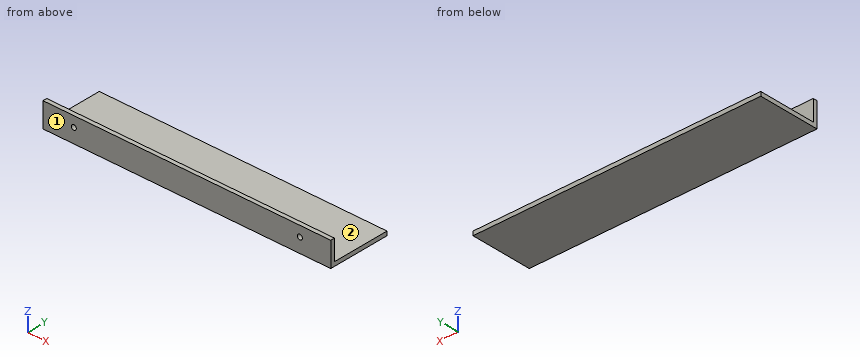
```python
from build123d import *

# Parameters (mm, degrees)
SZKIC1_W                    = 700
SZKIC1_H                    = 150
DODANIE_WYCI_GNI_CIE1_DEPTH = 10
SZKIC2_W                    = 700
SZKIC2_H                    = 10
DODANIE_WYCI_GNI_CIE2_DEPTH = 50
OTW_R_POD_RUB_M101_D        = 12
SZYK_LINIOWY2_COUNT         = 2
SZYK_LINIOWY2_PITCH         = 550


with BuildPart() as part:
    # Szkic1 → Dodanie-wyciągnięcie1 (new body)
    with BuildSketch(Plane.XY):
        Rectangle(SZKIC1_W, SZKIC1_H)
    extrude(amount=DODANIE_WYCI_GNI_CIE1_DEPTH)

    # Szkic2 → Dodanie-wyciągnięcie2 (add)
    with BuildSketch(Plane.XY.offset(10)):
        with Locations((0, -70)):
            Rectangle(SZKIC2_W, SZKIC2_H)
    extrude(amount=DODANIE_WYCI_GNI_CIE2_DEPTH)

    # Otwór pod śrubę M101 (through all)
    with Locations(Plane(origin=(0, -65, 0), x_dir=(1, 0, 0), z_dir=(0, 1, 0))):
        with Locations((-275, -35)):
            otw_r_pod_rub_m101 = Hole(OTW_R_POD_RUB_M101_D / 2)

    # Szyk liniowy2: Otwór pod śrubę M101 ×2
    with Locations(*[(i * SZYK_LINIOWY2_PITCH, 0, 0) for i in range(1, SZYK_LINIOWY2_COUNT)]):
        add(otw_r_pod_rub_m101, mode=Mode.SUBTRACT)


solid = part.part
```
Part model, mm, in its own coordinate system. Face numbers are marked on the shaded views. A direction names the side the tool comes from. Give positions to 0.01 mm unless a question says otherwise; leave off trailing zeros. Write each loop counter-clockwise with the first axis right and the second up, starting at its lowest first coordinate (ties: lowest second). Pieces come first, ordered by that corner, then holes. Notation, with made-up numbers: (-39, 72.25) -> (16, 72.25) arc R9 ccw to (16, 86.25) -> close; hole circle Ø9 at (-33.5, 63). An arc over 180 degrees is marked (long way). Put each result on its own line as item: value. Start each with the question number.
Item 1: Which spindle directions (+Z, -Z, +X, -X, +Y, -Y) get a long thin tool onto all of the face, cutting with end or side? Do the marked faces 1 and 2. Say none if no direction does.
Item 2: Cut at B-B (z = 35). List the corners of the cut face in (x, y), then the cut area to 3 significant figures.
Item 3: Wall check: L1, parallel to Z at x = 275, y = -67.75; L2, parallel to X at y = -69, z = 35; L3, parallel to Y at x = -83, z = 43.5. Give the ranges that are in metal, low to high. Write a range as [from, to].
Item 4: Cut at A-A (x = -275). List the corners of the cut face in (y, z), then the cut area to 3 significant figures.
Item 5: Cut at C-C (y = -7). List the corners of the cut face in (x, z).
Item 6: Cut at D-D (x = 38). List the corners of the cut face in (y, z).
Item 7: Pin check, flat tips, straight feed: pin 1 Ø25 at (x, z) = (-147, 31.5) entering from +Y; pin 2 Ø5 at (y, z) = (15.5, 13.5) entering from -X; pin 3 Ø1.5 at (x, y) = (-227, -13.5) entering from +Z. Stop position of each tip, or through.
Answer list:
1. face 1: +Z, -Z, +X, -X, -Y
1. face 2: +Z, +X, -X, +Y
2. outline: (-350, -75) -> (-281, -75) -> (-281, -65) -> (-350, -65) -> close; (-269, -75) -> (269, -75) -> (269, -65) -> (-269, -65) -> close; (281, -75) -> (350, -75) -> (350, -65) -> (281, -65) -> close
2. area: 6,760 mm2
3. L1: z = [0, 29], [41, 60]
3. L2: x = [-350, -281], [-269, 269], [281, 350]
3. L3: y = [-75, -65]
4. outline: (-75, 0) -> (75, 0) -> (75, 10) -> (-65, 10) -> (-65, 29) -> (-75, 29) -> close; (-75, 41) -> (-65, 41) -> (-65, 60) -> (-75, 60) -> close
4. area: 1,880 mm2
5. outline: (-350, 0) -> (350, 0) -> (350, 10) -> (-350, 10) -> close
6. outline: (-75, 0) -> (75, 0) -> (75, 10) -> (-65, 10) -> (-65, 60) -> (-75, 60) -> close
7. pin 1: stops at y = -65
7. pin 2: passes through
7. pin 3: stops at z = 10
